Autodesk Inventor part; units mm, degrees
ref_plane "YZ Plane" through (0, 0, 0) normal (1, 0, 0) x (0, 1, 0)
ref_plane "XZ Plane" through (0, 0, 0) normal (0, 1, 0) x (-1, 0, 0)
ref_plane "XY Plane" through (0, 0, 0) normal (0, 0, 1) x (1, 0, 0)
sketch "Sketch1" plane through (0, 0, 0) normal (0, 0, 1) x (1, 0, 0)
  line L0 (-12.7, -25.4) -> (12.7, -25.4)
  line L1 (12.7, -25.4) -> (12.7, 25.4)
  line L2 (12.7, 25.4) -> (-12.7, 25.4)
  line L3 (-12.7, 25.4) -> (-12.7, -25.4)
  line L4 (-12.7, -25.4) -> (12.7, 25.4) construction
  line L5 (12.7, -25.4) -> (-12.7, 25.4) construction
  point P0 (0, 0)
  dimension "d0" = 25.4
  dimension "d1" = 50.8
extrude "Extrusion1" add sketch "Sketch1" along normal blind 3.175
sketch "Sketch2" plane through (0, 0, 3.175) normal (0, 0, 1) x (1, 0, 0)
  line L0 (-12.7, -25.4) -> (12.7, -25.4)
  line L1 (12.7, 25.4) -> (-12.7, 25.4)
  line L2 (-12.7, 25.4) -> (-12.7, -25.4)
  line L3 (0, 25.4) -> (0, 12.7)
  line L4 (0, -25.4) -> (0, -12.7)
  point P0 (0, 0)
  dimension "d4" = 12.7
  dimension "d5" = 12.7
hole "Hole1" at (0, 12.7, 3.175) at (0, -12.7, 3.175) direction (0, 0, -1) diameter 6.35 end through all
properties part number "2 hole plate"
Geometry check sheet. Reference: the model listing, model coordinates, mm. Give positions to 0.01 mm unless a question says otherwise; leave off trailing zeros. Order: outer loops, then holes, each group sorted by start corner. A loop starts at its lowest first (then second) coordinate and runs counter-clockwise, first axis right, second up. Notation, with made-up numbers: (-20.5, 0) - (-12.5, 0) arc R23 cw to (-12.5, 31) - close; hole circle Ø4 at (30, 89.25). An arc over 180 degrees is marked (long way). Answer as a JSON object with one key per item and string values.
(1) Cross-section at C-C (z = 1.8). Record the cut outline in (x, y) (3 decimals), then the cut area to 3 significant figures.
Report:
{"outline": "(-12.7, -25.4) - (12.7, -25.4) - (12.7, 25.4) - (-12.7, 25.4) - close; hole circle Ø6.35 at (0, -12.7); hole circle Ø6.35 at (0, 12.7)", "area": "1,230 mm^2"}
(2) Cross-section at A-A (y = 12.7). Record the cut outline in (x, z) (3 decimals), then the cut area to 3 significant figures.
Report:
{"outline": "(-12.7, 0) - (-3.175, 0) - (-3.175, 3.175) - (-12.7, 3.175) - close; (3.175, 0) - (12.7, 0) - (12.7, 3.175) - (3.175, 3.175) - close", "area": "60.5 mm^2"}
(3) Depth check by flat-ended pin: pin 1 Ø5 at (x, y) = (0, 12.7) entering from -Z. Enter the tip coordinate at first touch or a pass-through.
Report:
{"pin 1": "through"}
(4) Cross-section at D-D (y = -12). Record the cut outline in (x, z) (3 decimals), then the cut area to 3 significant figures.
Report:
{"outline": "(-12.7, 0) - (-3.097, 0) - (-3.097, 3.175) - (-12.7, 3.175) - close; (3.097, 0) - (12.7, 0) - (12.7, 3.175) - (3.097, 3.175) - close", "area": "61.0 mm^2"}
(5) Cross-section at B-B (x = 0). Record the cut outline in (y, z) (3 decimals).
Report:
{"outline": "(-25.4, 0) - (-15.875, 0) - (-15.875, 3.175) - (-25.4, 3.175) - close; (-9.525, 0) - (9.525, 0) - (9.525, 3.175) - (-9.525, 3.175) - close; (15.875, 0) - (25.4, 0) - (25.4, 3.175) - (15.875, 3.175) - close"}
(6) Draft check along X on faces 1 (the flat face through (-12.7, 0, 2)), 2 (the flat face through (0, 0, 3.175)), 3 (the cylindrical face through (-0.95, 9.67, 1.57)). Enter one of: released by +X, released by -X, zero draft, split by the parting line, or undercut.
Report:
{"face 1": "released by -X", "face 2": "zero draft", "face 3": "undercut"}
(7) Material ranges on line 1 (Y direction, x = 0, z = 0.8) (3 decimals); line 2 (X direction, y = -12.7, z = 1.7) (3 decimals); line 3 (X direction, y = -11, z = 0.8), recorded low to high.
Report:
{"line 1": "-25.4 to -15.875, -9.525 to 9.525, 15.875 to 25.4", "line 2": "-12.7 to -3.175, 3.175 to 12.7", "line 3": "-12.7 to -2.68, 2.68 to 12.7"}
